Geometry check sheet. Reference: the model listing, model coordinates, mm. Face numbers are marked on the shaded views. A direction names the side the tool comes from. Round coordinates to 2 decimals unless told otherwise and drop trailing zeros. Loops run counter-clockwise (first coordinate to the right, second up) from the corner with the lowest first, then second, coordinate; pieces in that order, holes last.
```python
from build123d import *

# Parameters (mm, degrees)
SKETCH1_R                        = 4.03225
BOSS_EXTRUDE1_DEPTH              = 3.175
FILLET1_R                        = 12.7
EXTRUDE_THIN1_DEPTH              = 50.8
SKETCH3_W                        = 6.35
SKETCH3_H                        = 48.26
BOSS_EXTRUDE2_DEPTH              = 25.4
F_1_4_CLEARANCE_HOLE1_AT_2_COUNT = 2
F_1_4_CLEARANCE_HOLE1_AT_2_PITCH = 25.4
FILLET2_R                        = 6.35
FILLET3_R                        = 1.5875


with BuildPart() as part:
    # Sketch1 → Boss-Extrude1 (new, symmetric)
    with BuildSketch(Plane(origin=(0, 0, 0), x_dir=(1, 0, 0), z_dir=(0, 1, 0))):
        with BuildLine():
            Line((-25.4, 50.8), (25.4, 50.8))
            Line((25.4, 50.8), (25.4, 18.594090512))
            Line((25.4, 18.594090512), (10.998522628, -6.35))
            ThreePointArc((10.998522628, -6.35), (0, -12.7), (-10.998522628, -6.35))
            Line((-10.998522628, -6.35), (-25.4, 18.594090512))
            Line((-25.4, 18.594090512), (-25.4, 50.8))
        make_face()
        with Locations(Location((0, 0, 0), (0, 0, 270))):
            Circle(SKETCH1_R, mode=Mode.SUBTRACT)
    extrude(amount=BOSS_EXTRUDE1_DEPTH, both=True)

    # Fillet1
    fillet1_edges = [part.edges().sort_by_distance(p)[0] for p in [
        (25.4, 0, -18.594090512),
        (-25.4, 0, -18.594090512),
    ]]
    fillet(fillet1_edges, radius=FILLET1_R)

    # Sketch2 → Extrude-Thin1 (add)
    with BuildSketch(Plane(origin=(25.4, 0, 0), x_dir=(0, 0, -1), z_dir=(1, 0, 0))):
        Polygon((50.8, 3.175), (72.009, 3.175), (72.009, -4.445), (100.584, -4.445), (100.584, -52.705), (94.234, -52.705), (94.234, -10.795), (65.659, -10.795), (65.659, -3.175), (50.8, -3.175), align=None)
    extrude(amount=-EXTRUDE_THIN1_DEPTH)

    # Sketch3 → Boss-Extrude2 (add)
    with BuildSketch(Plane(origin=(25.4, 0, 0), x_dir=(0, 0, -1), z_dir=(1, 0, 0))):
        with Locations((97.409, -28.575)):
            Rectangle(SKETCH3_W, SKETCH3_H)
    boss_extrude2 = extrude(amount=BOSS_EXTRUDE2_DEPTH)

    # Sketch5 → 1/4 Clearance Hole1 (revolve, cut)
    with BuildSketch(Plane(origin=(41.275, -15.875, -94.234), x_dir=(0, -1, 0), z_dir=(1, 0, 0))):
        Polygon((0, 0), (0, 6.35), (4.0132, 6.35), (3.3782, 5.715), (3.3782, 0.635), (4.0132, 0), align=None)
    f_1_4_clearance_hole1 = revolve(axis=Axis((41.275, -15.875, -87.884), (0, 0, -1)), mode=Mode.SUBTRACT)

    # 1/4 Clearance Hole1 at 2: 1/4 Clearance Hole1 ×2
    with Locations(*[(0, -i * F_1_4_CLEARANCE_HOLE1_AT_2_PITCH, 0) for i in range(1, F_1_4_CLEARANCE_HOLE1_AT_2_COUNT)]):
        add(f_1_4_clearance_hole1, mode=Mode.SUBTRACT)

    # Mirror1: Boss-Extrude2, 1/4 Clearance Hole1 across plane
    add(boss_extrude2.mirror(Plane(origin=(0, 0, 0), x_dir=(0, 0, 1), z_dir=(1, 0, 0))))
    add(f_1_4_clearance_hole1.mirror(Plane(origin=(0, 0, 0), x_dir=(0, 0, 1), z_dir=(1, 0, 0))), mode=Mode.SUBTRACT)

    # Mirror1 copy 1 sketch → Mirror1 copy 1 (revolve, cut)
    with BuildSketch(Plane(origin=(-41.275, -41.275, -94.234), x_dir=(0, -1, 0), z_dir=(-1, 0, 0))):
        Polygon((0, 0), (0, -6.35), (4.0132, -6.35), (3.3782, -5.715), (3.3782, -0.635), (4.0132, 0), align=None)
    revolve(axis=Axis((-41.275, -41.275, -87.884), (0, 0, 1)), mode=Mode.SUBTRACT)

    # Fillet2
    fillet2_edges = [part.edges().sort_by_distance(p)[0] for p in [
        (25.4, -7.62, -94.234),
        (-25.4, -7.62, -94.234),
    ]]
    fillet(fillet2_edges, radius=FILLET2_R)

    # Fillet3
    fillet3_edges = [part.edges().sort_by_distance(p)[0] for p in [
        (0, -4.445, -72.009),
        (0, -3.175, -65.659),
        (0, -10.795, -65.659),
        (0, -10.795, -94.234),
    ]]
    fillet(fillet3_edges, radius=FILLET3_R)


solid = part.part
```
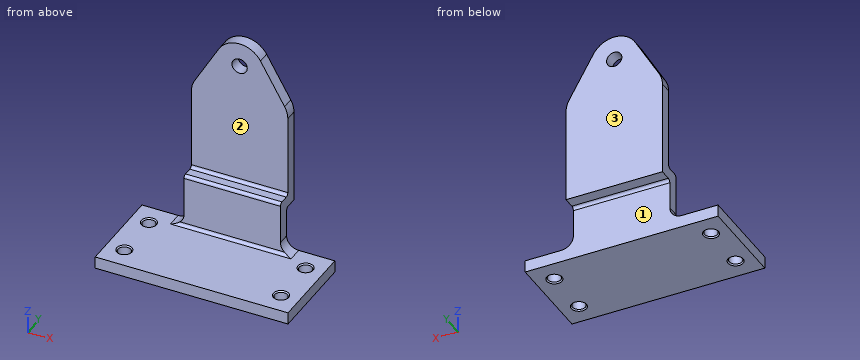
1) Scan lines: line 1 along Y through (x, z) = (-22.5, -83) (3 decimals); line 2 along Z through (x, y) = (-38, -35.5); line 3 along Y through (x, z) = (-20, -37.5) (3 decimals). Record each from-to range of solid material in increasing order.
Report:
line 1: y = -10.795 to -4.445
line 2: z = -100.58 to -94.23
line 3: y = -3.175 to 3.175
2) Sectioned sample at D-D, the plane z = -39. Record the cut outline in (x, y) (3 decimals), then the cut area to 3 significant figures.
Report:
outline: (-25.4, -3.175) - (25.4, -3.175) - (25.4, 3.175) - (-25.4, 3.175) - close
area: 323 mm2
3) Gauge pin test, flat ends, axial feed: pin 1 (6.5 mm diameter, centred on x = 9, y = 1.5, fed in from -Z); pin 2 (7.5 mm diameter, centred on x = 0, z = 0, fed in from +Y); pin 3 (7 mm diameter, centred on y = -3, z = -70, fed in from -X); pin 4 (2 mm diameter, centred on x = 6, y = -7, fed in from +Z). Record the tip position at first contact, or that the pin passes through.
Report:
pin 1: stops at z = -72.01
pin 2: passes through
pin 3: stops at x = -25.4
pin 4: stops at z = -65.66
4) Sectioned sample at C-C, the plane y = -6.5. Record the cut outline in (x, z), then the cut area to 3 significant figures.
Report:
outline: (-50.8, -100.58) - (50.8, -100.58) - (50.8, -94.23) - (31.75, -94.23) arc R6.35 cw to (25.4, -87.88) - (25.4, -65.66) - (-25.4, -65.66) - (-25.4, -87.88) arc R6.35 cw to (-31.75, -94.23) - (-50.8, -94.23) - close
area: 2,110 mm2
5) Access from +Z, -Z, +X, -X, +Y, -Y to the whole of each face (thin tool, end or side, straight path). Record for the marked faces 1, 2 and 3.
Report:
face 1: -Z, +X, -X, +Y
face 2: +Z, +X, -X, -Y
face 3: +Z, -Z, +X, -X, +Y
6) Sectioned sample at B-B, the plane x = 0. Record the cut outline in (y, z) (1 decimal).
Report:
outline: (-52.7, -100.6) - (-4.4, -100.6) - (-4.4, -73.6) arc R1.6 cw to (-2.9, -72) - (3.2, -72) - (3.2, -4) - (-3.2, -4) - (-3.2, -64.1) arc R1.6 cw to (-4.8, -65.7) - (-9.2, -65.7) arc R1.6 ccw to (-10.8, -67.2) - (-10.8, -92.6) arc R1.6 cw to (-12.4, -94.2) - (-52.7, -94.2) - close; (-3.2, 4) - (3.2, 4) - (3.2, 12.7) - (-3.2, 12.7) - close
7) Sectioned sample at A-A, the plane z = 0. Record the cut outline in (x, y) (3 decimals), then the cut area to 3 significant figures.
Report:
outline: (-14.665, -3.175) - (-4.032, -3.175) - (-4.032, 3.175) - (-14.665, 3.175) - close; (4.032, -3.175) - (14.665, -3.175) - (14.665, 3.175) - (4.032, 3.175) - close
area: 135 mm2
